```python
from build123d import *

# Parameters (mm, degrees)
BOSS_EXTRUDE1_DEPTH = 5


with BuildPart() as part:
    # Sketch2 → Boss-Extrude1 (new, symmetric)
    with BuildSketch(Plane.XY):
        with BuildLine():
            ThreePointArc((57, 17.916472867), (52.825722824, 12.985126011), (47.272727273, 16.287702607))
            ThreePointArc((47.272727273, 16.287702607), (0, 50), (-47.272727273, 16.287702607))
            ThreePointArc((-47.272727273, 16.287702607), (-52.825722824, 12.985126011), (-57, 17.916472867))
            Line((-57, 17.916472867), (-57, 30))
            ThreePointArc((-57, 30), (-72, 45), (-87, 30))
            Line((-87, 30), (-87, -30))
            ThreePointArc((-87, -30), (-72, -45), (-57, -30))
            Line((-57, -30), (-57, -17.916472867))
            ThreePointArc((-57, -17.916472867), (-52.825722824, -12.985126011), (-47.272727273, -16.287702607))
            ThreePointArc((-47.272727273, -16.287702607), (0, -50), (47.272727273, -16.287702607))
            ThreePointArc((47.272727273, -16.287702607), (52.825722824, -12.985126011), (57, -17.916472867))
            Line((57, -17.916472867), (57, -30))
            ThreePointArc((57, -30), (72, -45), (87, -30))
            Line((87, -30), (87, 30))
            ThreePointArc((87, 30), (72, 45), (57, 30))
            Line((57, 30), (57, 17.916472867))
        make_face()
        with BuildLine():
            Line((62, -30), (62, 30))
            ThreePointArc((62, 30), (72, 40), (82, 30))
            Line((82, 30), (82, -30))
            ThreePointArc((82, -30), (72, -40), (62, -30))
        make_face(mode=Mode.SUBTRACT)
        with BuildLine():
            ThreePointArc((-62, 30), (-72, 40), (-82, 30))
            Line((-82, 30), (-82, -30))
            ThreePointArc((-82, -30), (-72, -40), (-62, -30))
            Line((-62, -30), (-62, 30))
        make_face(mode=Mode.SUBTRACT)
        with BuildLine():
            ThreePointArc((24.348067415, -5.672002568), (24.692208515, 3.910861626), (21.403642989, 12.918361615))
            Line((21.403642989, 12.918361615), (33.636517601, 25.151236226))
            ThreePointArc((33.636517601, 25.151236226), (29.69848481, 29.69848481), (25.151236226, 33.636517601))
            Line((25.151236226, 33.636517601), (12.918361615, 21.403642989))
            ThreePointArc((12.918361615, 21.403642989), (3.910861626, 24.692208515), (-5.672002568, 24.348067415))
            Line((-5.672002568, 24.348067415), (-13.525991536, 39.762388673))
            ThreePointArc((-13.525991536, 39.762388673), (-19.067600989, 37.422274016), (-24.218069826, 34.314502676))
            Line((-24.218069826, 34.314502676), (-16.364080859, 18.900181419))
            ThreePointArc((-16.364080859, 18.900181419), (-22.275163105, 11.349762493), (-24.90913336, 2.129571608))
            Line((-24.90913336, 2.129571608), (-41.996040101, -0.576728553))
            ThreePointArc((-41.996040101, -0.576728553), (-41.482910305, -6.570247532), (-40.118826521, -12.42898864))
            Line((-40.118826521, -12.42898864), (-23.03191978, -9.722688479))
            ThreePointArc((-23.03191978, -9.722688479), (-17.67766953, -17.67766953), (-9.722688479, -23.03191978))
            Line((-9.722688479, -23.03191978), (-12.42898864, -40.118826521))
            ThreePointArc((-12.42898864, -40.118826521), (-6.570247532, -41.482910305), (-0.576728553, -41.996040101))
            Line((-0.576728553, -41.996040101), (2.129571608, -24.90913336))
            ThreePointArc((2.129571608, -24.90913336), (11.349762493, -22.275163105), (18.900181419, -16.364080859))
            Line((18.900181419, -16.364080859), (34.314502676, -24.218069826))
            ThreePointArc((34.314502676, -24.218069826), (37.422274016, -19.067600989), (39.762388673, -13.525991536))
            Line((39.762388673, -13.525991536), (24.348067415, -5.672002568))
        make_face(mode=Mode.SUBTRACT)
    extrude(amount=BOSS_EXTRUDE1_DEPTH, both=True)


solid = part.part
```
Geometry check sheet. Reference: the model listing, model coordinates, mm. A direction names the side the tool comes from. Give positions to 0.01 mm unless a question says otherwise; leave off trailing zeros. Write each loop counter-clockwise with the first axis right and the second up, starting at its lowest first coordinate (ties: lowest second). Pieces come first, ordered by that corner, then holes. Notation, with made-up numbers: (-29, 65) -> (15, 65) arc R9 cw to (15, 70) -> close; hole circle Ø10 at (88, 33.25). An arc over 180 degrees is marked (long way). Use one line per item in the form item = value.
Item 1: Scan lines: line 1 (X direction, y = 3, z = -3.5); line 2 (X direction, y = 35, z = -0.5); line 3 (X direction, y = 4, z = -0.5). Record each from-to range of solid material in increasing order.
Results list:
line_1 = -87 to -82, -62 to -24.82, 24.82 to 62, 82 to 87
line_2 = -86.14 to -80.66, -63.34 to -57.86, -35.71 to -23.22, -11.1 to 35.71, 57.86 to 63.34, 80.66 to 86.14
line_3 = -87 to -82, -62 to -24.68, 24.68 to 62, 82 to 87
Item 2: Sectioned sample at A-A on x = 72. Enter the section's corners in (y, z), plus the area to 3 significant figures.
Results list:
outline = (-45, -5) -> (-40, -5) -> (-40, 5) -> (-45, 5) -> close; (40, -5) -> (45, -5) -> (45, 5) -> (40, 5) -> close
area = 100 mm2
Item 3: Sectioned sample at D-D on z = 2.75. Count the separate pieces of the cut face and the enclosed holes in it, plus the area to 3 significant figures.
Results list:
separate_pieces = 1
enclosed_holes = 3
area = 7,270 mm2
Item 4: Sectioned sample at C-C on y = 37. Enter the section's corners in (x, z).
Results list:
outline = (-85.27, -5) -> (-79.14, -5) -> (-79.14, 5) -> (-85.27, 5) -> close; (-64.86, -5) -> (-58.73, -5) -> (-58.73, 5) -> (-64.86, 5) -> close; (-33.63, -5) -> (-19.87, -5) -> (-19.87, 5) -> (-33.63, 5) -> close; (-12.12, -5) -> (33.63, -5) -> (33.63, 5) -> (-12.12, 5) -> close; (58.73, -5) -> (64.86, -5) -> (64.86, 5) -> (58.73, 5) -> close; (79.14, -5) -> (85.27, -5) -> (85.27, 5) -> (79.14, 5) -> close
Item 5: Mould release check, pull along X, two halves, no side actions. Record for faces 4 (the cylindrical face through (-18.99, 37.46, 0.07)), 5 (the flat face through (-21, -22, 5)), 6 (the flat face through (87, 0, 0)), 7 (the cylindrical face through (-72, 40, 0)): released by +X, released by -X, zero draft, split by the parting line, or undercut.
Results list:
face_4 = undercut
face_5 = zero draft
face_6 = released by +X
face_7 = undercut
Item 6: Depth check by flat-ended pin: pin 1 Ø3 at (x, z) = (-46.5, -0.5) entering from -Y. Enter the tip coordinate at first touch or a pass-through.
Results list:
pin_1 = -21.79
Item 7: Access from +Z, -Z, +X, -X, +Y, -Y to the whole of each face (thin tool, end or side, straight path). Record for faces 1 (the cylindrical face through (29.758, 29.639, 0.07)), 2 (the flat face through (57, 24, 0)), 3 (the flat face through (-57, -24, 0)).
Results list:
face_1 = +Z, -Z
face_2 = +Z, -Z, +Y
face_3 = +Z, -Z, -Y
Item 8: Sectioned sample at B-B on y = 7. Enter the section's corners in (x, z).
Results list:
outline = (-87, -5) -> (-82, -5) -> (-82, 5) -> (-87, 5) -> close; (-62, -5) -> (-24, -5) -> (-24, 5) -> (-62, 5) -> close; (24, -5) -> (62, -5) -> (62, 5) -> (24, 5) -> close; (82, -5) -> (87, -5) -> (87, 5) -> (82, 5) -> close
